Build history of the part. All positions in model axes, mm. Face numbers are marked on the shaded views. A direction names the side the tool comes from. Give positions to 0.01 mm unless a question says otherwise; leave off trailing zeros. Order: outer loops, then holes, each group sorted by start corner. A loop starts at its lowest first (then second) coordinate and runs counter-clockwise, first axis right, second up. Notation, with made-up numbers: (-11, 7.5) - (-1, 7.5) arc R32 cw to (-1, 42.5) - close; hole circle Ø1 at (-15, 73). An arc over 180 degrees is marked (long way). One line per item, written item: value.
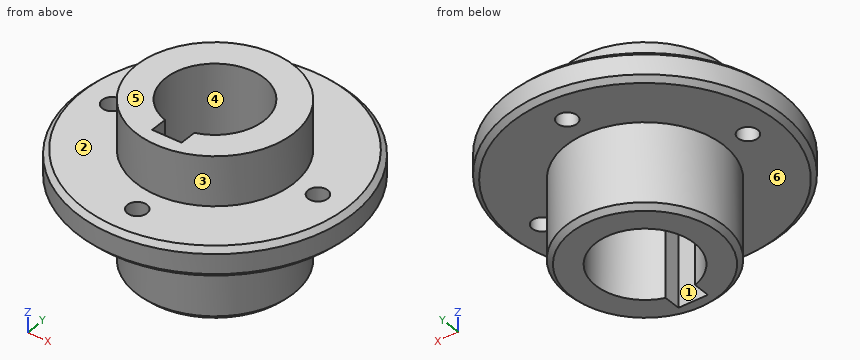
```python
from build123d import *

# Parameters (mm, degrees)
SKETCH_1_R               = 16
EXTRUDE_1_DEPTH          = 13
SKETCH_2_R               = 16
EXTRUDE_2_DEPTH          = 4
SKETCH_3_R               = 28
EXTRUDE_3_DEPTH          = 6
SKETCH_4_R               = 7
EXTRUDE_4_DEPTH          = 5
SKETCH_6_R               = 2
CUT_EXTRUDE_1_DEPTH      = 10
SKETCH_7_R               = 10
CUT_EXTRUDE_2_DEPTH      = 60
PATTERN_CIRCULAR_2_COUNT = 4
CHAMFER_3_SIZE           = 1
CHAMFER_4_SIZE           = 1
CHAMFER_6_SIZE           = 1
SKETCH_8_R               = 16
SKETCH_8_R_2             = 10
EXTRUDE_5_DEPTH          = 10
CUT_EXTRUDE_3_DEPTH      = 13


with BuildPart() as part:
    # 草图1 → 凸台-拉伸1 (new body)
    with BuildSketch(Plane.XY):
        with Locations(Location((0, 0, 0), (0, 0, 180))):
            Circle(SKETCH_1_R)
    extrude(amount=EXTRUDE_1_DEPTH)

    # 草图2 → 凸台-拉伸2 (add)
    with BuildSketch(Plane.XY.offset(13)):
        with Locations(Location((0, 0, 0), (0, 0, 180))):
            Circle(SKETCH_2_R)
    extrude(amount=EXTRUDE_2_DEPTH)

    # 草图3 → 凸台-拉伸3 (add)
    with BuildSketch(Plane.XY.offset(17)):
        Circle(SKETCH_3_R)
    extrude(amount=EXTRUDE_3_DEPTH)

    # 草图4 → 凸台-拉伸4 (add)
    with BuildSketch(Plane.XY.offset(23)):
        Circle(SKETCH_4_R)
    extrude(amount=EXTRUDE_4_DEPTH)

    # 草图6 → 切除-拉伸1 (cut)
    with BuildSketch(Plane(origin=(0, 0, 17), x_dir=(-1, 0, 0), z_dir=(0, 0, -1))):
        with Locations((0, 21)):
            Circle(SKETCH_6_R)
    cut_extrude_1 = extrude(amount=-CUT_EXTRUDE_1_DEPTH, mode=Mode.SUBTRACT)

    # 草图7 → 切除-拉伸2 (cut)
    with BuildSketch(Plane(origin=(0, 0, 0), x_dir=(-1, 0, 0), z_dir=(0, 0, -1))):
        Circle(SKETCH_7_R)
    extrude(amount=-CUT_EXTRUDE_2_DEPTH, mode=Mode.SUBTRACT)

    # 阵列(圆周)2: 切除-拉伸1 ×4 about axis
    pattern_circular_2_axis = Axis((0, 0, 0), (0, 0, 1))
    for i in range(1, PATTERN_CIRCULAR_2_COUNT):
        add(cut_extrude_1.rotate(pattern_circular_2_axis, i * 360 / PATTERN_CIRCULAR_2_COUNT), mode=Mode.SUBTRACT)

    # 倒角3
    chamfer_3_edges = [part.edges().sort_by_distance(p)[0] for p in [
        (-28, 0, 23),
    ]]
    chamfer(chamfer_3_edges, length=CHAMFER_3_SIZE)

    # 倒角4
    chamfer_4_edges = [part.edges().sort_by_distance(p)[0] for p in [
        (-28, 0, 17),
    ]]
    chamfer(chamfer_4_edges, length=CHAMFER_4_SIZE)

    # 倒角6
    chamfer_6_edges = [part.edges().sort_by_distance(p)[0] for p in [
        (16, 0, 0),
    ]]
    chamfer(chamfer_6_edges, length=CHAMFER_6_SIZE)

    # 草图8 → 凸台-拉伸5 (add)
    with BuildSketch(Plane.XY.offset(23)):
        with Locations(Location((0, 0, 0), (0, 0, 180))):
            Circle(SKETCH_8_R)
        with Locations(Location((0, 0, 0), (0, 0, 180))):
            Circle(SKETCH_8_R_2, mode=Mode.SUBTRACT)
    extrude(amount=EXTRUDE_5_DEPTH)

    # 草图9 → 切除-拉伸3 (cut)
    with BuildSketch(Plane(origin=(0, 0, 0), x_dir=(1, 0, 0), z_dir=(0, 1, 0))):
        Polygon((-3, 0), (0, 0), (3, 0), (3, -33), (-3, -33), align=None)
    extrude(amount=-CUT_EXTRUDE_3_DEPTH, mode=Mode.SUBTRACT)


solid = part.part
```
(1) Slice it at A-A, the plane y = 0. Count the separate pieces of the cut face and the enclosed holes in it, and give its area (3 significant figures).
Completed:
separate pieces: 4
enclosed holes: 0
area: 489 mm²
(2) Drill centre lines: line 1 (Z direction, x = 13.5, y = -18); line 2 (Y direction, x = -4.5, z = 4); line 3 (X direction, y = -11.5, z = 29). Where is each one in solid material? Low to high.
Completed:
line 1: 17 to 23
line 2: -15.35 to -8.93, 8.93 to 15.35
line 3: -11.12 to -3, 3 to 11.12
(3) 3-axis set-ups, long thin cutter, end or side, ignore diameter. For the marked faces 5 and 6: which of +Z, -Z, +X, -X, +Y, -Y reach the whole face in a straight line?
Completed:
face 5: +Z, +X, -X, +Y, -Y
face 6: -Z
(4) Slice it at B-B, the plane z = 28. Give the cut face in (x, y).
Completed:
outline: circle Ø32 at (0, 0); hole (-3, -13) - (3, -13) - (3, -9.54) arc R10 ccw (long way) to (-3, -9.54) - close
(5) Pin check, flat tips, straight feed: P1, Ø5, axis at x = 0, y = -21, coming from the +Z side; P2, Ø1.7, axis at y = -11.5, z = 21, coming from the -X side; P3, Ø6.5, axis at x = -1, z = 16, coming from the +Y side. Stop position of each tip, or through.
Completed:
P1: z = 23
P2: x = -25.9
P3: y = 28
(6) Pull direction X, two halves, no side cores. Call the marked faces 1, 2, 3 and 4: +X half, -X half, draft (parallel to the pull), parting line (faces both ways), or undercut.
Completed:
face 1: undercut
face 2: draft
face 3: parting line
face 4: undercut
